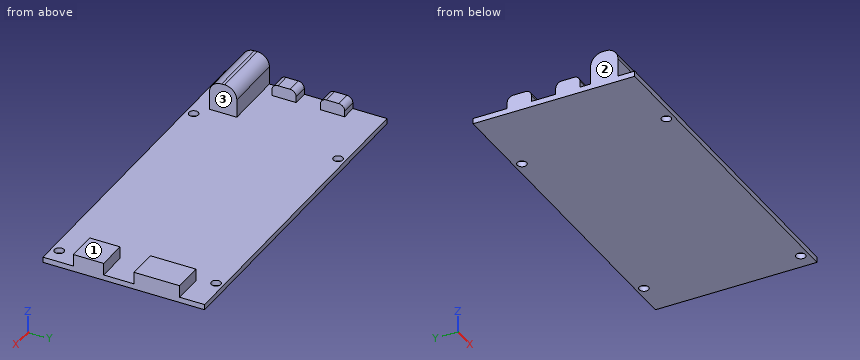
Autodesk Inventor part; units mm, degrees
ref_plane "YZ Plane" through (0, 0, 0) normal (1, 0, 0) x (0, 1, 0)
ref_plane "XZ Plane" through (0, 0, 0) normal (0, 1, 0) x (-1, 0, 0)
ref_plane "XY Plane" through (0, 0, 0) normal (0, 0, 1) x (1, 0, 0)
sketch "Sketch1" plane through (0, 0, 0) normal (0, 0, 1) x (1, 0, 0)
  line L0 (11.35, 0) -> (123.35, 0)
  line L1 (123.35, 0) -> (123.35, 53.25)
  line L2 (123.35, 53.25) -> (11.35, 53.25)
  line L3 (11.35, 53.25) -> (11.35, 0)
  line L4 (13.2018, 50.8) -> (120.6255, 50.8) construction
  line L5 (12.1008, 2.54) -> (119.6818, 2.54) construction
  point P0 (0, 0)
  point P1 (0, 0)
  point P2 (36.84, 50.8)
  point P3 (111.77, 50.8)
  point P4 (118.12, 2.54)
  point P5 (35.57, 2.54)
  dimension "d0" = 112
  dimension "d1" = 53.25
  dimension "d2" = 48.26
  dimension "d3" = 2.45
  dimension "d4" = 74.93
  dimension "d5" = 82.55
  dimension "d6" = 6.35
  dimension "d7" = 5.23
  dimension "d38" = 100.42
  dimension "d39" = 1.27
extrude "Extrusion1" add sketch "Sketch1" along normal blind 1.8
hole "Hole1" at (36.84, 50.8, 0) at (111.77, 50.8, 0) at (118.12, 2.54, 0) at (35.57, 2.54, 0) direction (0, 0, 1) diameter 3.1 end through all
sketch "Sketch2" plane through (0, 0, 1.8) normal (0, 0, 1) x (1, 0, 0)
  line L0 (123.35, 0) -> (123.35, 53.25)
  line L1 (123.35, 10) -> (113.35, 10)
  line L2 (113.35, 10) -> (113.35, 20)
  line L3 (113.35, 20) -> (123.35, 20)
  line L4 (123.35, 20) -> (123.35, 10)
  line L5 (11.35, 0) -> (123.35, 0)
  line L6 (123.35, 45) -> (113.35, 45)
  line L7 (113.35, 45) -> (113.35, 30)
  line L8 (113.35, 30) -> (123.35, 30)
  line L9 (123.35, 30) -> (123.35, 45)
  line L10 (11.35, 53.25) -> (11.35, 0)
  line L11 (11.35, 5.5) -> (31.35, 5.5)
  line L12 (31.35, 5.5) -> (31.35, 14.5)
  line L13 (31.35, 14.5) -> (11.35, 14.5)
  line L14 (11.35, 14.5) -> (11.35, 5.5)
  line L15 (11.35, 42) -> (16.35, 42)
  line L16 (16.35, 42) -> (16.35, 34)
  line L17 (16.35, 34) -> (11.35, 34)
  line L18 (11.35, 34) -> (11.35, 42)
  line L19 (11.35, 26) -> (16.35, 26)
  line L20 (16.35, 26) -> (16.35, 18)
  line L21 (16.35, 18) -> (11.35, 18)
  line L22 (11.35, 18) -> (11.35, 26)
  point P0 (0, 0)
  dimension "d17" = 10
  dimension "d18" = 10
  dimension "d19" = 10
  dimension "d20" = 10
  dimension "d21" = 15
  dimension "d22" = 30
  dimension "d23" = 20
  dimension "d24" = 9
  dimension "d25" = 5
  dimension "d26" = 8
  dimension "d27" = 5
  dimension "d28" = 8
  dimension "d29" = 5.5
  dimension "d30" = 18
  dimension "d31" = 34
extrude "Extrusion2" add sketch "Sketch2" along normal blind 4
extrude "Extrusion3" add sketch "Sketch2" along normal blind 10 contours L10 L13 L12 L11
fillet "Fillet1" radius 4 2 edges at (21.35, 14.5, 11.8) (21.35, 5.5, 11.8)
fillet "Fillet2" radius 2 4 edges at (13.85, 26, 5.8) (13.85, 18, 5.8) (13.85, 34, 5.8) (13.85, 42, 5.8)
properties part number "EVAL_ADICUP360"
The listing builds one solid part. Answer for the finished solid, in the listing's coordinates (mm). Face numbers are marked on the shaded views. Round coordinates to 2 decimals unless told otherwise and drop trailing zeros. Order: outer loops, then holes, each group sorted by start corner. A loop starts at its lowest first (then second) coordinate and runs counter-clockwise, first axis right, second up. Notation, with made-up numbers: M 73.25,-11.75 L 122.25,-11.75 A10 cw 122.25,3.25 Z; hole C -18,-17 d11. An arc over 180 degrees is marked long. Answer in a Markdown table with one row per item. Add a question column.
1) The part is cut by section C-C on y = 38. Determine the outline of the cut face in (x, z), plus the area to 3 significant figures.
2) Determine the mould class of the marked faces 1, 2 and 3 for opening direction X: pulls with the +X half, pulls with the -X half, needs draft (parallel to the pull), parting line crosses it, or undercut.
3) The part is cut by section D-D on x = 20. Determine the outline of the cut face in (y, z), plus the area to 3 significant figures.
4) Flat-ended cylindrical pins translate along their axes: pin 1 Ø1.6 at (x, z) = (15, 3) entering from -Y; pin 2 Ø1 at (x, z) = (15, 2.5) entering from +Y; pin 3 Ø4 at (x, y) = (118.12, 2.54) entering from +Z. Find the tip coordinate at first contact, or state that the pin passes through.
5) The part is cut by section B-B on x = 111.77. Determine the outline of the cut face in (y, z), plus the area to 3 significant figures.
6) Consider line 1 along X through (y, z) = (50.8, 0.4); line 2 along X through (y, z) = (2.54, 1.4); line 3 along X through (y, z) = (36.5, 2.75). Determine where each line is inside the solid, lowest interval first. Write a range as from..to.
7) The part is cut by section A-A on y = 2.54. Determine the outline of the cut face in (x, z), plus the area to 3 significant figures.
Findings below:
| question | item | result |
|---|---|---|
| 1 | outline | M 11.35,0 L 123.35,0 L 123.35,5.8 L 113.35,5.8 L 113.35,1.8 L 16.35,1.8 L 16.35,5.8 L 11.35,5.8 Z |
| 1 | area | 262 mm² |
| 2 | face 1 | needs draft |
| 2 | face 2 | pulls with the -X half |
| 2 | face 3 | undercut |
| 3 | outline | M 0,0 L 53.25,0 L 53.25,1.8 L 14.5,1.8 L 14.5,7.8 A4 ccw 10.5,11.8 L 9.5,11.8 A4 ccw 5.5,7.8 L 5.5,1.8 L 0,1.8 Z |
| 3 | area | 179 mm² |
| 4 | pin 1 | stops at y = 5.5 |
| 4 | pin 2 | stops at y = 42 |
| 4 | pin 3 | stops at z = 1.8 |
| 5 | outline | M 0,0 L 49.25,0 L 49.25,1.8 L 0,1.8 Z; M 52.35,0 L 53.25,0 L 53.25,1.8 L 52.35,1.8 Z |
| 5 | area | 90.3 mm² |
| 6 | line 1 | x = 11.35..35.29, 38.39..110.22, 113.32..123.35 |
| 6 | line 2 | x = 11.35..34.02, 37.12..116.57, 119.67..123.35 |
| 6 | line 3 | x = 11.35..16.35, 113.35..123.35 |
| 7 | outline | M 11.35,0 L 34.02,0 L 34.02,1.8 L 11.35,1.8 Z; M 37.12,0 L 116.57,0 L 116.57,1.8 L 37.12,1.8 Z; M 119.67,0 L 123.35,0 L 123.35,1.8 L 119.67,1.8 Z |
| 7 | area | 190 mm² |
